Input: part model. Units: mm. Frame: model coordinates. A direction names the side the tool comes from. Give positions to 0.01 mm unless a question says otherwise; leave off trailing zeros. Order: outer loops, then holes, each group sorted by start corner. A loop starts at its lowest first (then second) coordinate and runs counter-clockwise, first axis right, second up. Notation, with made-up numbers: M 38,41 L 91,41 A20 ccw 91,78 Z; hole C 15.5,69.5 d2. An arc over 180 degrees is marked long. Use a Markdown table: item, result.
from build123d import *

# Parameters (mm, degrees)
SKETCH1_W             = 40
SKETCH1_H             = 26
ESC_BODY_DEPTH        = 5
SKETCH2_R             = 2.38125
MOTOR_WIRES_DEPTH     = 12.7
SKETCH3_R             = 3.81
CAPACITOR_HEADS_DEPTH = 6.35
SKETCH4_R             = 2.38125
POWER_WIRES_DEPTH     = 12.7
FILLET1_R             = 2.54


with BuildPart() as part:
    # Sketch1 → ESC Body (new, symmetric)
    with BuildSketch(Plane(origin=(0, 0, 0), x_dir=(1, 0, 0), z_dir=(0, 1, 0))):
        Rectangle(SKETCH1_W, SKETCH1_H)
    extrude(amount=ESC_BODY_DEPTH, both=True)

    # Sketch2 → Motor Wires (add)
    with BuildSketch(Plane(origin=(20, 0, 0), x_dir=(0, 0, -1), z_dir=(1, 0, 0))):
        with Locations(Location((0, 0, 0), (0, 0, 180))):
            Circle(SKETCH2_R)
        with Locations(Location((-9.525, 0, 0), (0, 0, 180))):
            Circle(SKETCH2_R)
        with Locations(Location((9.525, 0, 0), (0, 0, 180))):
            Circle(SKETCH2_R)
    extrude(amount=MOTOR_WIRES_DEPTH)

    # Sketch3 → Capacitor Heads (add)
    with BuildSketch(Plane.ZY.offset(20)):
        with Locations(Location((-4.064, 0, 0), (0, 0, 180))):
            Circle(SKETCH3_R)
        with Locations(Location((4.064, 0, 0), (0, 0, 180))):
            Circle(SKETCH3_R)
    extrude(amount=CAPACITOR_HEADS_DEPTH)

    # Sketch4 → Power Wires (add)
    with BuildSketch(Plane.ZY.offset(20)):
        with Locations(Location((-10.61875, 0, 0), (0, 0, 180))):
            Circle(SKETCH4_R)
        with Locations((10.61875, 0)):
            Circle(SKETCH4_R)
    extrude(amount=POWER_WIRES_DEPTH)

    # Fillet1
    fillet1_edges = [part.edges().sort_by_distance(p)[0] for p in [
        (0, 5, 13),
        (0, -5, 13),
        (0, -5, -13),
        (0, 5, -13),
    ]]
    fillet(fillet1_edges, radius=FILLET1_R)


solid = part.part
1) Material intervals for line 1 (Z direction, x = 23, y = -1); line 2 (X direction, y = -0.5, z = -2); line 3 (Z direction, x = -22, y = -1.5), sorted ascending. Write a range as from..to.
Response values:
| item | result |
|---|---|
| line 1 | z = -11.69..-7.36, -2.16..2.16, 7.36..11.69 |
| line 2 | x = -26.35..32.7 |
| line 3 | z = -12.47..-8.77, -7.57..-0.56, 0.56..7.57, 8.77..12.47 |
2) First-contact query: pin 1 Ø2.5 at (y, z) = (0, 4) entering from -X. Flat tip, straight axial feed; report the tip coordinate or a pass-through.
Response values:
| item | result |
|---|---|
| pin 1 | stops at x = -26.35 |
3) Cut plane A-A on x = -21.5. Return loops of the section in (y, z).
Response values:
| item | result |
|---|---|
| outline | C 0,-4.06 d7.62; C 0,4.06 d7.62; C 0,-10.62 d4.76; C 0,10.62 d4.76 |
4) Reachability of faces 5 (the face through (-26.35, 0, 4)), 6 (the face through (-23.13, -1.14, 0.43)), 7 (the face through (32.7, 0, 9)), 8 (the face through (20, 0, 3)), 9 (the face through (-32.7, 0, 11)) from +Z, -Z, +X, -X, +Y, -Y: full face, straight path, thin tool, end or side. Return the list, or none.
Response values:
| item | result |
|---|---|
| face 5 | -X, +Y, -Y |
| face 6 | -X |
| face 7 | +Z, -Z, +X, +Y, -Y |
| face 8 | +X |
| face 9 | +Z, -Z, -X, +Y, -Y |
5) Cut plane C-C on x = 1.5. Return loops of the section in (y, z).
Response values:
| item | result |
|---|---|
| outline | M -5,-10.46 A2.54 ccw -2.46,-13 L 2.46,-13 A2.54 ccw 5,-10.46 L 5,10.46 A2.54 ccw 2.46,13 L -2.46,13 A2.54 ccw -5,10.46 Z |
6) Mould query, pull axis Z, two halves, no side actions, for faces 1 (the face through (32.7, 0, -10)), 2 (the face through (26.261, -0.105, 7.146)), 3 (the face through (0.28, -4.236, -12.276)), 4 (the face through (0.28, 4.236, 12.276)). Classes: released by +Z, released by -Z, zero draft, split by the parting line, or undercut.
Response values:
| item | result |
|---|---|
| face 1 | zero draft |
| face 2 | undercut |
| face 3 | released by -Z |
| face 4 | released by +Z |
7) Cut plane B-B on z = -6.25. Return loops of the section in (x, y).
Response values:
| item | result |
|---|---|
| outline | M -26.35,-3.12 L -20,-3.12 L -20,-5 L 20,-5 L 20,5 L -20,5 L -20,3.12 L -26.35,3.12 Z |
